Geometry check sheet. Reference: the model listing, model coordinates, mm. Face numbers are marked on the shaded views. A direction names the side the tool comes from. Give positions to 0.01 mm unless a question says otherwise; leave off trailing zeros. Order: outer loops, then holes, each group sorted by start corner. A loop starts at its lowest first (then second) coordinate and runs counter-clockwise, first axis right, second up.
from build123d import *

# Parameters (mm, degrees)
F0_W     = 25.4
F0_H     = 19.05
F0_H_2   = 4.7498
F0_H_3   = 4.7752
F1_DEPTH = 25.4


with BuildPart() as f1:
    # F0 (on Front) → F1 (new body, symmetric)
    with BuildSketch(Plane.XZ):
        Polygon((85.725, 66.675), (85.725, 61.9252), (85.725, 42.8752), (85.725, 38.1), (111.125, 38.1), (111.125, 66.675), align=None)
        with Locations((73.025, 52.4002)):
            Rectangle(F0_W, F0_H)
        with Locations((73.025, 64.3001)):
            Rectangle(F0_W, F0_H_2)
        with Locations((73.025, 40.4876)):
            Rectangle(F0_W, F0_H_3)
        with BuildLine():
            Line((22.225, 27.0002), (22.225, 9.525))
            Line((22.225, 9.525), (41.275, 9.525))
            Line((41.275, 9.525), (41.275, 27.0002))
            ThreePointArc((41.275, 27.0002), (45.9246798487, 38.2255201513), (57.15, 42.8752))
            Line((57.15, 42.8752), (60.325, 42.8752))
            Line((60.325, 42.8752), (60.325, 61.9252))
            Line((60.325, 61.9252), (57.15, 61.9252))
            ThreePointArc((57.15, 61.9252), (32.4542956671, 51.6959043329), (22.225, 27.0002))
        make_face()
    extrude(amount=F1_DEPTH, both=True)


solid = f1.part
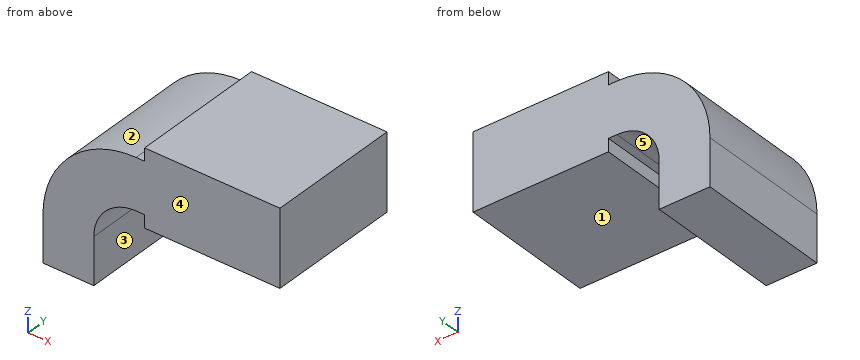
Item 1: Sectioned sample at B-B (y = -10). Enter the section's corners in (x, z) (3 decimals), and give its area (3 significant figures).
Reported:
outline: (22.225, 9.525) - (41.275, 9.525) - (41.275, 27) arc R15.875 cw to (57.15, 42.875) - (60.325, 42.875) - (60.325, 38.1) - (111.125, 38.1) - (111.125, 66.675) - (60.325, 66.675) - (60.325, 61.925) - (57.15, 61.925) arc R34.925 ccw to (22.225, 27) - close
area: 2,610 mm2
Item 2: Sectioned sample at C-C (x = 74.5). Enter the section's corners in (y, z) (3 decimals).
Reported:
outline: (-25.4, 38.1) - (25.4, 38.1) - (25.4, 66.675) - (-25.4, 66.675) - close
Item 3: Scan lines: L1, parallel to Z at x = 105.5, y = 13.5 (3 decimals); L2, parallel to X at y = -16, z = 18 (3 decimals); L3, parallel to Z at x = 55, y = -10. Record each from-to range of solid material in increasing order.
Reported:
L1: z = 38.1 to 66.675
L2: x = 22.225 to 41.275
L3: z = 42.73 to 61.86
Item 4: Gauge pin test, flat ends, axial feed: pin 1 (2.5 mm diameter, centred on x = 59, y = 0.5, fed in from -Z); pin 2 (2 mm diameter, centred on y = -5, z = 37.5, fed in from -X); pin 3 (8 mm diameter, centred on y = 2.5, z = 22, fed in from +X) (3 decimals). Record the tip position at first contact, or that the pin passes through.
Reported:
pin 1: stops at z = 42.88
pin 2: stops at x = 23.54
pin 3: stops at x = 41.275
Item 5: Sectioned sample at D-D (z = 22). Enter the section's corners in (x, y) (3 decimals).
Reported:
outline: (22.225, -25.4) - (41.275, -25.4) - (41.275, 25.4) - (22.225, 25.4) - close
Item 6: Draft check along X on the marked faces 3, 4 and 5. Enter one of: released by +X, released by -X, zero draft, split by the parting line, or undercut.
Reported:
face 3: released by +X
face 4: zero draft
face 5: undercut
Item 7: Sectioned sample at A-A (z = 41.5). Enter the section's corners in (x, y) (3 decimals).
Reported:
outline: (25.377, -25.4) - (50.687, -25.4) - (50.687, 25.4) - (25.377, 25.4) - close; (60.325, -25.4) - (111.125, -25.4) - (111.125, 25.4) - (60.325, 25.4) - close
Item 8: Set-up check for the marked faces 1 and 2: record each of +Z, -Z, +X, -X, +Y, -Y from which the full face is reachable in a straight line by a thin tool's end or side.
Reported:
face 1: -Z, +X, +Y, -Y
face 2: +Z, -X, +Y, -Y
